The model under review builds one solid part; all positions refer to its coordinate system, in mm. A direction names the side the tool comes from. Coordinates: 2 decimals unless noted, no trailing zeros. Order: outer loops, then holes, each group sorted by start corner. A loop starts at its lowest first (then second) coordinate and runs counter-clockwise, first axis right, second up. Notation, with made-up numbers: M 70.25,4.5 L 105.25,4.5 A29 ccw 105.25,37.5 Z; hole C 0.25,60 d9. An arc over 180 degrees is marked long. Answer in a Markdown table with one row per item.
from build123d import *

# Parameters (mm, degrees)
SKETCH1_R           = 60
SKETCH1_R_2         = 54
SKETCH1_R_3         = 8
BOSS_EXTRUDE1_DEPTH = 3
SKETCH1_3_R         = 8
BOSS_EXTRUDE2_DEPTH = 5
CUT_EXTRUDE1_REACH  = 10
SKETCH2_R           = 1.5
CUT_EXTRUDE2_REACH  = 5
SKETCH3_R           = 3.75
SKETCH4_R           = 1.5
CUT_EXTRUDE3_DEPTH  = 5


with BuildPart() as part:
    # Sketch1 → Boss-Extrude1 (new body)
    with BuildSketch(Plane(origin=(0, 0, 0), x_dir=(1, 0, 0), z_dir=(0, 1, 0))):
        Circle(SKETCH1_R)
        Circle(SKETCH1_R_2, mode=Mode.SUBTRACT)
        with BuildLine():
            ThreePointArc((7.5, -53.47663041), (3.660460389, -52.338407931), (2.000000204, -48.694167705))
            Line((2.000000204, -48.694167705), (2.000000204, -16.899494443))
            ThreePointArc((2.000000204, -16.899494443), (3.134156671, -11.197704847), (6.363961031, -6.363961031))
            ThreePointArc((6.363961031, -6.363961031), (11.197704847, -3.134156671), (16.899494443, -2.000000204))
            Line((16.899494443, -2.000000204), (48.694167705, -2.000000204))
            ThreePointArc((48.694167705, -2.000000204), (52.338407931, -3.660460389), (53.47663041, -7.5))
            ThreePointArc((53.47663041, -7.5), (53.868998701, -3.759119436), (54, 0))
            ThreePointArc((54, 0), (53.868998701, 3.759119436), (53.47663041, 7.5))
            ThreePointArc((53.47663041, 7.5), (52.338407931, 3.660460389), (48.694167705, 2.000000204))
            Line((48.694167705, 2.000000204), (16.899494443, 2.000000204))
            ThreePointArc((16.899494443, 2.000000204), (11.197704847, 3.134156671), (6.363961031, 6.363961031))
            ThreePointArc((6.363961031, 6.363961031), (3.134156671, 11.197704847), (2.000000204, 16.899494443))
            Line((2.000000204, 16.899494443), (2.000000204, 48.694167705))
            ThreePointArc((2.000000204, 48.694167705), (3.660460389, 52.338407931), (7.5, 53.47663041))
            ThreePointArc((7.5, 53.47663041), (0, 54), (-7.5, 53.47663041))
            ThreePointArc((-7.5, 53.47663041), (-3.660460389, 52.338407931), (-2.000000204, 48.694167705))
            Line((-2.000000204, 48.694167705), (-2.000000204, 16.899494443))
            ThreePointArc((-2.000000204, 16.899494443), (-3.134156671, 11.197704847), (-6.363961031, 6.363961031))
            ThreePointArc((-6.363961031, 6.363961031), (-11.197704847, 3.134156671), (-16.899494443, 2.000000204))
            Line((-16.899494443, 2.000000204), (-48.694167705, 2.000000204))
            ThreePointArc((-48.694167705, 2.000000204), (-52.338407931, 3.660460389), (-53.47663041, 7.5))
            ThreePointArc((-53.47663041, 7.5), (-54, 0), (-53.47663041, -7.5))
            ThreePointArc((-53.47663041, -7.5), (-52.338407931, -3.660460389), (-48.694167705, -2.000000204))
            Line((-48.694167705, -2.000000204), (-16.899494443, -2.000000204))
            ThreePointArc((-16.899494443, -2.000000204), (-11.197704847, -3.134156671), (-6.363961031, -6.363961031))
            ThreePointArc((-6.363961031, -6.363961031), (-3.134156671, -11.197704847), (-2.000000204, -16.899494443))
            Line((-2.000000204, -16.899494443), (-2.000000204, -48.694167705))
            ThreePointArc((-2.000000204, -48.694167705), (-3.660460389, -52.338407931), (-7.5, -53.47663041))
            ThreePointArc((-7.5, -53.47663041), (0, -54), (7.5, -53.47663041))
        make_face()
        Circle(SKETCH1_R_3, mode=Mode.SUBTRACT)
        Circle(SKETCH1_R_3)
    extrude(amount=-BOSS_EXTRUDE1_DEPTH)

    # Sketch1_3 → Boss-Extrude2 (add)
    with BuildSketch(Plane(origin=(0, 0, 0), x_dir=(1, 0, 0), z_dir=(0, 1, 0))):
        Circle(SKETCH1_3_R)
    extrude(amount=BOSS_EXTRUDE2_DEPTH)

    # Sketch2 → Cut-Extrude1 (cut, up to next)
    with BuildSketch(Plane(origin=(0, 5, 0), x_dir=(1, 0, 0), z_dir=(0, 1, 0)), mode=Mode.PRIVATE) as cut_extrude1_sk1:
        Circle(SKETCH2_R)
    cut_extrude1_tool1 = extrude(cut_extrude1_sk1.sketch, amount=-CUT_EXTRUDE1_REACH, mode=Mode.PRIVATE) & part.part
    add(cut_extrude1_tool1.solids().sort_by_distance((0, 5, 0))[0], mode=Mode.SUBTRACT)

    # Sketch3 → Cut-Extrude2 (cut, up to next)
    with BuildSketch(Plane(origin=(0, 0, 0), x_dir=(1, 0, 0), z_dir=(0, 1, 0)), mode=Mode.PRIVATE) as cut_extrude2_sk1:
        with Locations((0, -55.25)):
            Circle(SKETCH3_R)
    cut_extrude2_tool1 = extrude(cut_extrude2_sk1.sketch, amount=-CUT_EXTRUDE2_REACH, mode=Mode.PRIVATE) & part.part
    add(cut_extrude2_tool1.solids().sort_by_distance((0, 0, 55.25))[0], mode=Mode.SUBTRACT)

    # Sketch4 → Cut-Extrude3 (cut)
    with BuildSketch(Plane(origin=(0, 5, 0), x_dir=(1, 0, 0), z_dir=(0, 1, 0))):
        with Locations((0, -5.5)):
            Circle(SKETCH4_R)
    extrude(amount=-CUT_EXTRUDE3_DEPTH, mode=Mode.SUBTRACT)


solid = part.part
(1) Take a section at C-C (z = 11). Write out the cut boundary in (x, y).
Report:
| item | result |
|---|---|
| outline | M -58.98,-3 L -52.87,-3 L -52.87,0 L -58.98,0 Z; M -3.22,-3 L 3.22,-3 L 3.22,0 L -3.22,0 Z; M 52.87,-3 L 58.98,-3 L 58.98,0 L 52.87,0 Z |
(2) Take a section at A-A (y = -1.5). Write out the cut boundary in (x, z).
Report:
| item | result |
|---|---|
| outline | C 0,0 d120; hole M -53.48,-7.5 A54 ccw -7.5,-53.48 A4.83 ccw -2,-48.69 L -2,-16.9 A14.9 ccw -16.9,-2 L -48.69,-2 A4.83 ccw Z; hole M -53.48,7.5 A4.83 ccw -48.69,2 L -16.9,2 A14.9 ccw -2,16.9 L -2,48.69 A4.83 ccw -7.5,53.48 A54 ccw Z; hole C 0,55.25 d7.5; hole C 0,0 d3; hole M 2,-48.69 A4.83 ccw 7.5,-53.48 A54 ccw 53.48,-7.5 A4.83 ccw 48.69,-2 L 16.9,-2 A14.9 ccw 2,-16.9 Z; hole M 2,16.9 A14.9 ccw 16.9,2 L 48.69,2 A4.83 ccw 53.48,7.5 A54 ccw 7.5,53.48 A4.83 ccw 2,48.69 Z |
(3) Insertion check: P1, Ø4, axis at x = -5.5, z = -27, coming from the -Y side; P2, Ø0.9, axis at y = -1.5, z = -32.5, coming from the +X side; P3, Ø1.5, axis at y = -1, z = 29.5, coming from the -X side; P4, Ø1, axis at x = 3.5, y = -1, coming from the +Z side. Each pin has a flat end and moves straight along its axis. Give the tip position at first contact, or say it passes through.
Report:
| item | result |
|---|---|
| P1 | through |
| P2 | x = 50.72 |
| P3 | x = -52.66 |
| P4 | z = 59.92 |
(4) Take a section at B-B (x = 0). Write out the cut boundary in (y, z), then the cut area to 4 significant figures.
Report:
| item | result |
|---|---|
| outline | M -3,-60 L 0,-60 L 0,-8 L 5,-8 L 5,-1.5 L -3,-1.5 Z; M -3,1.5 L 5,1.5 L 5,4 L 0,4 L 0,7 L 5,7 L 5,8 L 0,8 L 0,51.5 L -3,51.5 Z; M -3,59 L 0,59 L 0,60 L -3,60 Z |
| area | 378.5 mm^2 |
(5) Take a section at D-D (z = 55.25). Write out the cut boundary in (x, y).
Report:
| item | result |
|---|---|
| outline | M -23.4,-3 L -3.75,-3 L -3.75,0 L -23.4,0 Z; M 3.75,-3 L 23.4,-3 L 23.4,0 L 3.75,0 Z |
(6) Machinability: for faces 5 (the flat face through (0, -3, 4)), 6 (the flat face through (-2, -1, 33)), 7 (the flat face through (0, 0, 5)), which of the approach directions +Z, -Z, +X, -X, +Y, -Y give a long, thin tool a straight path to every point of the face, cutting with its end or side? Answer none if there is none.
Report:
| item | result |
|---|---|
| face 5 | +Z, -Z, +X, -X, -Y |
| face 6 | +Y, -Y |
| face 7 | +Y |
(7) The part is to be moulded in two halves that separate along X. For faces 1 (the cylindrical face through (3.704, -1.479, 52.376)), 2 (the cylindrical face through (-59.94, -1.48, -2.64)), 3 (the flat face through (2, 5, 0)), 4 (the flat face through (2, -1, 33)), say which applies: +X half, -X half, draft (parallel to the pull), parting line (faces both ways), or undercut.
Report:
| item | result |
|---|---|
| face 1 | undercut |
| face 2 | parting line |
| face 3 | draft |
| face 4 | undercut |
(8) To check wall thickness, follow line 1 (Z direction, x = 0, y = -1); line 2 (X direction, y = -0.5, z = 0); line 3 (X direction, y = -0.75, z = 17). State the ranges of each line that lie inside material, in increasing order. Write a range as [from, to].
Report:
| item | result |
|---|---|
| line 1 | [-60, -1.5], [1.5, 51.5], [59, 60] |
| line 2 | [-60, -1.5], [1.5, 60] |
| line 3 | [-57.54, -51.25], [-2, 2], [51.25, 57.54] |
